Autodesk Inventor part; units mm, degrees
ref_plane "YZ Plane" through (0, 0, 0) normal (1, 0, 0) x (0, 1, 0)
ref_plane "XZ Plane" through (0, 0, 0) normal (0, 1, 0) x (-1, 0, 0)
ref_plane "XY Plane" through (0, 0, 0) normal (0, 0, 1) x (1, 0, 0)
sketch "Sketch1" plane through (0, 0, 0) normal (0, 1, 0) x (-1, 0, 0)
  circle A0 centre (0, 0) radius 10.541
  dimension "d2" = 21.082
extrude "Extrusion1" add sketch "Sketch1" along normal blind 2.032
sketch "Sketch2" plane through (0, 0, 0) normal (0, -1, 0) x (1, 0, 0)
  circle A0 centre (0, 0) radius 10.541
  circle A1 centre (0, 0) radius 9.017
  dimension "d4" = 18.034
extrude "Extrusion2" add sketch "Sketch2" along normal blind 24.003 contours A1
hole "Hole1" at (0, 2.032, 0) direction (0, -1, 0) diameter 13.97 end through all
ref_plane "Work Plane1" through (0, -13.6652, 0) normal (0, 1, 0) x (1, 0, 0)
sketch "Sketch3" plane through (0, -13.6652, 0) normal (0, 1, 0) x (1, 0, 0)
  line L0 (0, 0) -> (9.017, 0)
  line L1 (9.017, 0) -> (9.017, -9.017)
  line L2 (9.017, -9.017) -> (0, -9.017)
  line L3 (0, -9.017) -> (0, 0)
  dimension "d17" = 9.017
  dimension "d18" = 9.017
extrude "Extrusion3" cut sketch "Sketch3" along normal blind 3.175
sketch "Sketch4" plane through (0, 2.032, 0) normal (0, 1, 0) x (1, 0, 0)
  circle A0 centre (0, 0) radius 10.541
  circle A1 centre (7.62, -6.35) radius 0.508
  line L0 (7.62, -6.35) -> (0, 0) construction
  line L1 (7.9452, -5.9597) -> (8.4136, -6.3501)
  line L2 (7.2948, -6.7403) -> (7.7632, -7.1306)
  dimension "d21" = 1.016
  dimension "d22" = 6.35
  dimension "d23" = 7.62
extrude "Extrusion4" cut sketch "Sketch4" against normal up to surface (2.032 mm away) contours L2 A1 L1 A0 | A1 picked at (8.2446, -6.4771)
properties part number "Piston Shaft" material "Stainless Steel"
The listing builds one solid part. Answer for the finished solid, in the listing's coordinates (mm). A direction names the side the tool comes from. Coordinates: 2 decimals unless noted, no trailing zeros. Order: outer loops, then holes, each group sorted by start corner. A loop starts at its lowest first (then second) coordinate and runs counter-clockwise, first axis right, second up. Notation, with made-up numbers: M 44.25,-6 L 98.25,-6 A11 ccw 98.25,1 Z; hole C -26.5,12 d8. An arc over 180 degrees is marked long. Answer as a JSON object with one key per item and string values. Group by question number.
1. Section C-C on x = -5.25 is taken. Write down the section's boundary in (y, z), then the cut area to 3 significant figures.
2. Straight lines are drawn through the part: line 1 (Z direction, x = 0, y = -9) (3 decimals); line 2 (Z direction, x = -3.75, y = -15.25); line 3 (X direction, y = -1.25, z = 5.25). For each, find the intervals that lie inside material, in ascending order.
3. A tool of negligible diameter and unlimited length cuts with its end or side. For faces 4 (the cylindrical face through (-6.65, -11.83, -6.09)), 5 (the flat face through (0, -12, 8)), 6 (the cylindrical face through (-4.72, -11.17, -5.15)), from which of +Z, -Z, +X, -X, +Y, -Y can it reach the whole face along a straight path? Write none if from no direction.
4. Determine the mould class of faces 1 (the cylindrical face through (7.237, 1.03, 6.016)), 2 (the flat face through (-7, 2.032, -2)), 3 (the flat face through (8, -12, 0)) for opening direction Y: released by +Y, released by -Y, zero draft, split by the parting line, or undercut.
5. Section D-D on y = -9.5 is taken. Write down the section's boundary in (x, z) (3 decimals), then the cut area to 3 significant figures.
6. Flat-ended cylindrical pins translate along their axes: P1, Ø1, axis at y = -12.5, z = 7.5, coming from the +X side; P2, Ø0.6, axis at x = 7.5, y = -11.5, coming from the +Z side; P3, Ø6, axis at y = -14, z = -0.5, coming from the -X side; P4, Ø4.5, axis at x = 5.5, z = 3, coming from the +Y side. Find the tip coordinate at first contact, or state that the pin passes through.
7. Section A-A on x = 1 is taken. Write down the section's boundary in (y, z), then the cut area to 3 significant figures.
8. Section B-B on z = 2.25 is taken. Write down the section's boundary in (x, y).
Values follow:
{
 "1": {"outline": "M -24,-7.33 L 0,-7.33 L 0,-9.14 L 2.03,-9.14 L 2.03,-4.61 L -24,-4.61 Z; M -24,4.61 L 2.03,4.61 L 2.03,9.14 L 0,9.14 L 0,7.33 L -24,7.33 Z", "area": "149 mm2"},
 "2": {"line 1": "-9.017 to -6.985, 6.985 to 9.017", "line 2": "-8.2 to -5.89, 5.89 to 8.2", "line 3": "-7.33 to -4.61, 4.61 to 7.33"},
 "3": {"face 4": "-Y", "face 5": "+Z, +X", "face 6": "+Y, -Y"},
 "4": {"face 1": "zero draft", "face 2": "released by +Y", "face 3": "undercut"},
 "5": {"outline": "C 0,0 d18.034; hole C 0,0 d13.97", "area": "102 mm2"},
 "6": {"P1": "x = 0", "P2": "z = 0", "P3": "x = -9.02", "P4": "y = 2.03"},
 "7": {"outline": "M -24,-8.96 L 0,-8.96 L 0,-10.49 L 2.03,-10.49 L 2.03,-6.91 L -24,-6.91 Z; M -24,6.91 L -13.67,6.91 L -13.67,8.96 L -24,8.96 Z; M -10.49,6.91 L 2.03,6.91 L 2.03,10.49 L 0,10.49 L 0,8.96 L -10.49,8.96 Z", "area": "106 mm2"},
 "8": {"outline": "M -10.3,0 L -8.73,0 L -8.73,-24 L -6.61,-24 L -6.61,2.03 L -10.3,2.03 Z; M 6.61,-24 L 8.73,-24 L 8.73,-13.67 L 6.61,-13.67 Z; M 6.61,-10.49 L 8.73,-10.49 L 8.73,0 L 10.3,0 L 10.3,2.03 L 6.61,2.03 Z"}
}
